Source: CAD feature listing. Evaluate the final solid. Frame: model axes, mm. Give positions to 0.01 mm unless a question says otherwise; leave off trailing zeros. Loops run counter-clockwise (first coordinate to the right, second up) from the corner with the lowest first, then second, coordinate; pieces in that order, holes last. Notation, with made-up numbers: (37.5, 82) -> (48.5, 82) arc R4 cw to (48.5, 86) -> close; hole circle Ø3 at (43.25, 70). An arc over 180 degrees is marked (long way). Return JSON: item names as keys, results as strings. Group by question number.
(1) Ray query, line 1 (X direction, y = 0.5, z = 2); line 2 (Y direction, x = -51, z = 2.4); line 3 (Y direction, x = -1.5, z = 0.7). Return the intervals inside material, ascending. Write a range as from..to.
(2) Cut plane B-B on y = 0. Return loops of the section in (x, z).
(3) Pin query (flat end, axial travel): pin 1 (4.5 mm diameter, centred on x = -71.12, y = 0, fed in from +Z); pin 2 (5.5 mm diameter, centred on x = -50.29, y = 50.29, fed in from +Z); pin 3 (1 mm diameter, centred on y = 21, z = 2, fed in from +X); pin 4 (1 mm diameter, centred on y = 20.5, z = 1, fed in from +X). Return the tip coordinate at first contact, or that it passes through.
(4) Cut plane D-D on y = -31. Return loops of the section in (x, z).
(5) Cut plane A-A on x = 9.5. Return loops of the section in (y, z).
(6) Cut plane C-C on z = 0.55. Return loops of the section in (x, y), then the cut area to 3 significant figures.
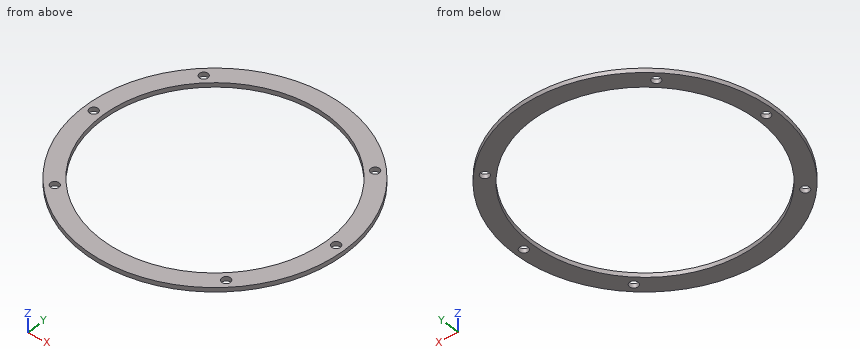
```python
from build123d import *

# Parameters (mm, degrees)
SKETCH1_R                  = 76.2
SKETCH1_R_2                = 66.04
BOSS_EXTRUDE1_DEPTH        = 2.54
F_10_CLEARANCE_HOLE1_D     = 4.9784
F_10_CLEARANCE_HOLE1_DEPTH = 38.354
F_10_CLEARANCE_HOLE1_TIP   = 1.495662253


with BuildPart() as part:
    # Sketch1 → Boss-Extrude1 (new body)
    with BuildSketch(Plane.XY):
        Circle(SKETCH1_R)
        Circle(SKETCH1_R_2, mode=Mode.SUBTRACT)
    extrude(amount=BOSS_EXTRUDE1_DEPTH)

    # #10 Clearance Hole1
    with Locations(Plane.XY.offset(2.54)):
        with Locations((-50.289434278, 50.289434278), (-71.12, 0), (-50.289434278, -50.289434278), (50.289434278, -50.289434278), (71.12, 0), (50.289434278, 50.289434278)):
            Hole(F_10_CLEARANCE_HOLE1_D / 2, depth=F_10_CLEARANCE_HOLE1_DEPTH)
            with Locations((0, 0, -(F_10_CLEARANCE_HOLE1_DEPTH + F_10_CLEARANCE_HOLE1_TIP / 2))):  # 118° drill point
                Cone(0, F_10_CLEARANCE_HOLE1_D / 2, F_10_CLEARANCE_HOLE1_TIP, mode=Mode.SUBTRACT)


solid = part.part
```
Answers:
{
 "1": {"line 1": "-76.2..-73.56, -68.68..-66.04, 66.04..68.68, 73.56..76.2", "line 2": "-56.62..-52.68, -47.9..-41.96, 41.96..47.9, 52.68..56.62", "line 3": "-76.19..-66.02, 66.02..76.19"},
 "2": {"outline": "(-76.2, 0) -> (-73.61, 0) -> (-73.61, 2.54) -> (-76.2, 2.54) -> close; (-68.63, 0) -> (-66.04, 0) -> (-66.04, 2.54) -> (-68.63, 2.54) -> close; (66.04, 0) -> (68.63, 0) -> (68.63, 2.54) -> (66.04, 2.54) -> close; (73.61, 0) -> (76.2, 0) -> (76.2, 2.54) -> (73.61, 2.54) -> close"},
 "3": {"pin 1": "through", "pin 2": "z = 2.54", "pin 3": "x = 73.39", "pin 4": "x = 73.53"},
 "4": {"outline": "(-69.61, 0) -> (-58.31, 0) -> (-58.31, 2.54) -> (-69.61, 2.54) -> close; (58.31, 0) -> (69.61, 0) -> (69.61, 2.54) -> (58.31, 2.54) -> close"},
 "5": {"outline": "(-75.61, 0) -> (-65.35, 0) -> (-65.35, 2.54) -> (-75.61, 2.54) -> close; (65.35, 0) -> (75.61, 0) -> (75.61, 2.54) -> (65.35, 2.54) -> close"},
 "6": {"outline": "circle Ø152.4 at (0, 0); hole circle Ø4.98 at (-71.12, 0); hole circle Ø132.08 at (0, 0); hole circle Ø4.98 at (-50.29, -50.29); hole circle Ø4.98 at (-50.29, 50.29); hole circle Ø4.98 at (50.29, -50.29); hole circle Ø4.98 at (50.29, 50.29); hole circle Ø4.98 at (71.12, 0)", "area": "4,420 mm²"}
}
